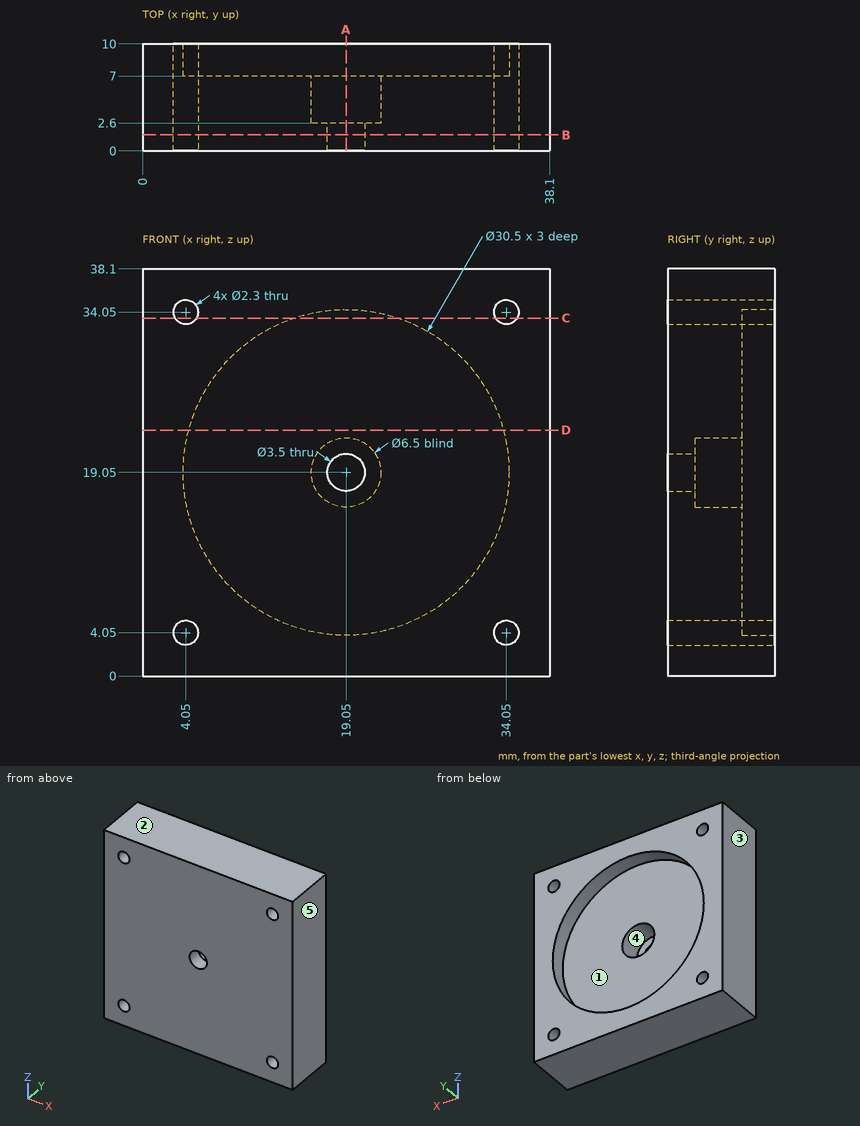
Can you work these out from the drawing? Everything is in mm from the part's minimum corner. A direction names the side the tool comes from. Round coordinates to 2 decimals unless told otherwise and drop trailing zeros. Loops run counter-clockwise (first coordinate to the right, second up) from the corner with the lowest first, then second, coordinate; pieces in that order, holes last. Notation, with made-up numbers: (48.25, 37.25) - (71.25, 37.25) arc R17 ccw to (71.25, 54.25) - close; hole circle Ø1 at (64.25, 9). An arc over 180 degrees is marked (long way). Answer in a Markdown table with one row per item. Add a question column.
Q1. I want a section at D-D on z = 23. List the corners of the cut face in (x, y) for me.
Q2. I need wall thicknesses on L1, parallel to Z at x = 34.05, y = 5.5; L2, parallel to Z at x = 19.05, y = 4.9; L3, parallel to Z at x = 19.05, y = 7.7. Which ranges of each line are inside material? Lowest first, please.
Q3. Which directions (+Z, -Z, +X, -X, +Y, -Y) give clear straight access to the entire face, cutting with the end or side of a thin tool? Please do the marked faces 4 and 5.
Q4. I want a section at A-A on x = 19.05. List the corners of the cut face in (y, z) for me.
Q5. I want a section at C-C on z = 33.5. List the corners of the cut face in (x, y) for me.
Q6. For pin 1 Ø7 at (x, z) = (18, 19) entering from +Y; pin 2 Ø4 at (x, z) = (19.05, 19.05) entering from +Y, each with a flat end and sliding along its axis, tell me the tip position at first contact or that it passes through.
Q7. We'd pull the mould along X, two halves only. Please class the marked faces 1, 2 and 3: pulls with the +X half, pulls with the -X half, needs draft (parallel to the pull), parting line crosses it, or undercut.
Q8. I want a section at B-B on y = 1.5. List the corners of the cut face in (x, z) for me.
A:
| question | item | result |
|---|---|---|
| 1 | outline | (0, 0) - (38.1, 0) - (38.1, 10) - (33.78, 10) - (33.78, 7) - (4.32, 7) - (4.32, 10) - (0, 10) - close |
| 2 | L1 | 0 to 2.9, 5.2 to 32.9, 35.2 to 38.1 |
| 2 | L2 | 0 to 15.8, 22.3 to 38.1 |
| 2 | L3 | 0 to 3.8, 34.3 to 38.1 |
| 3 | face 4 | +Y |
| 3 | face 5 | +Z, -Z, +X, +Y, -Y |
| 4 | outline | (0, 0) - (10, 0) - (10, 3.8) - (7, 3.8) - (7, 15.8) - (2.6, 15.8) - (2.6, 17.3) - (0, 17.3) - close; (0, 20.8) - (2.6, 20.8) - (2.6, 22.3) - (7, 22.3) - (7, 34.3) - (10, 34.3) - (10, 38.1) - (0, 38.1) - close |
| 5 | outline | (0, 0) - (3.04, 0) - (3.04, 10) - (0, 10) - close; (5.06, 0) - (33.04, 0) - (33.04, 10) - (23.92, 10) - (23.92, 7) - (14.18, 7) - (14.18, 10) - (5.06, 10) - close; (35.06, 0) - (38.1, 0) - (38.1, 10) - (35.06, 10) - close |
| 6 | pin 1 | y = 7 |
| 6 | pin 2 | y = 2.6 |
| 7 | face 1 | undercut |
| 7 | face 2 | needs draft |
| 7 | face 3 | pulls with the -X half |
| 8 | outline | (0, 0) - (38.1, 0) - (38.1, 38.1) - (0, 38.1) - close; hole circle Ø2.3 at (4.05, 4.05); hole circle Ø2.3 at (4.05, 34.05); hole circle Ø3.5 at (19.05, 19.05); hole circle Ø2.3 at (34.05, 4.05); hole circle Ø2.3 at (34.05, 34.05) |
